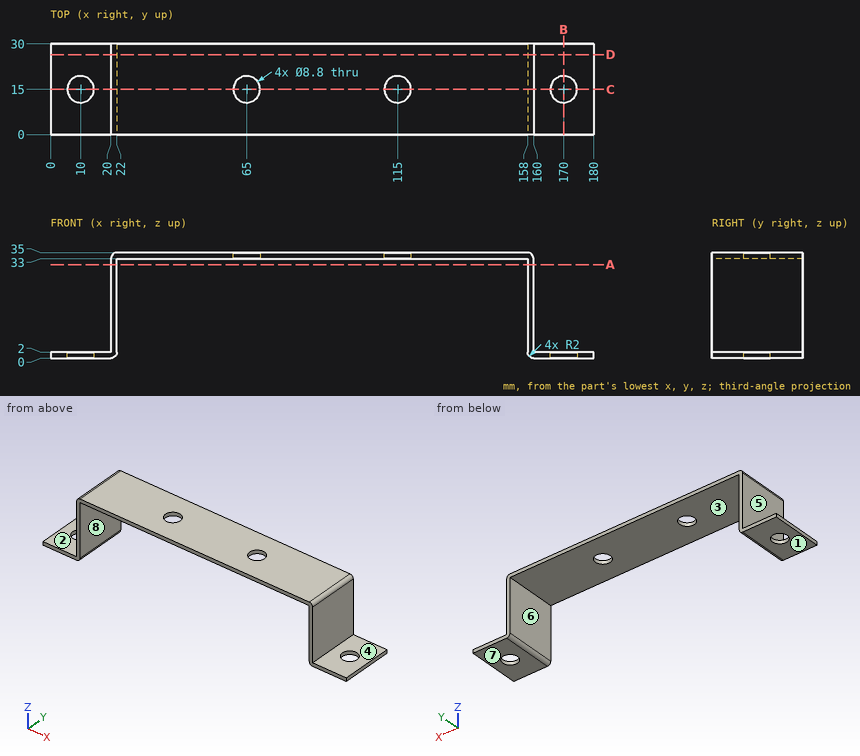
The figure shows three views and two pictorial views of one solid part (mm, origin at its lowest corner). Answer the questions. A direction names the side the tool comes from. Round coordinates to 2 decimals unless told otherwise and drop trailing zeros. Loops run counter-clockwise (first coordinate to the right, second up) from the corner with the lowest first, then second, coordinate; pieces in that order, holes last. Notation, with made-up numbers: M -21.5,-36.75 L 25.5,-36.75 A31 cw 25.5,-12.75 Z; hole C 59,-19 d7. An arc over 180 degrees is marked long. Write each question's results on one line, items separated by ' | '. Start each with the question number.
1) Which of the six approach directions +Z, -Z, +X, -X, +Y, -Y give full straight-line access (tool end or side, diameter ignored) to the marked faces 1, 2, 3 and 4?
2) Find section C-C on y = 15. Count the separate pieces of the cut face and the enclosed holes in it, plus the area to 3 significant figures.
3) Find section A-A on z = 31. Write down the section's boundary in (x, y), plus the area to 3 significant figures.
4) Find section D-D on y = 26.5. Write down the section's boundary in (x, z).
5) Find section B-B on x = 170. Write down the section's boundary in (y, z), plus the area to 3 significant figures.
6) Determine the mould class of the marked faces 5, 6, 7 and 8 for opening direction X: pulls with the +X half, pulls with the -X half, needs draft (parallel to the pull), parting line crosses it, or undercut.
7) Straight lines are drawn through the part: probe 1 along Y at (x, z) = (115, 33.6); probe 2 along X at (y, z) = (10, 21); probe 3 along Z at (x, y) = (84.5, 12.75). For each, find the intervals that lie inside material, in ascending order.
8) Each of these flat-tipped pins is pushed along its axis until it touches: pin 1 (7 mm diameter, centred on x = 10, y = 15, fed in from +Z); pin 2 (15 mm diameter, centred on x = 80.5, y = 19, fed in from -Z); pin 3 (2 mm diameter, centred on y = 22.5, z = 25.5, fed in from +X); pin 4 (16 mm diameter, centred on x = 8, y = 11.5, fed in from +Z). Where does it stop, or does it pass through?
Final values:
1) face 1: -Z, +X, -X, +Y, -Y | face 2: +Z, -X, +Y, -Y | face 3: -Z, +Y, -Y | face 4: +Z, +X, +Y, -Y
2) separate pieces: 5 | enclosed holes: 0 | area: 418 mm²
3) outline: M 20,0 L 22,0 L 22,30 L 20,30 Z; M 158,0 L 160,0 L 160,30 L 158,30 Z | area: 120 mm²
4) outline: M 0,0 L 20,0 A2 ccw 22,2 L 22,33 L 158,33 L 158,2 A2 ccw 160,0 L 180,0 L 180,2 L 160,2 L 160,33 A2 ccw 158,35 L 22,35 A2 ccw 20,33 L 20,2 L 0,2 Z
5) outline: M 0,0 L 10.6,0 L 10.6,2 L 0,2 Z; M 19.4,0 L 30,0 L 30,2 L 19.4,2 Z | area: 42.4 mm²
6) face 5: pulls with the -X half | face 6: undercut | face 7: needs draft | face 8: undercut
7) probe 1: 0 to 10.6, 19.4 to 30 | probe 2: 20 to 22, 158 to 160 | probe 3: 33 to 35
8) pin 1: through | pin 2: z = 33 | pin 3: x = 160 | pin 4: z = 2
